Geometry: final body of the model. Coordinates: model frame, mm. Face numbers are marked on the shaded views. Give positions to 0.01 mm unless a question says otherwise; leave off trailing zeros. Write each loop counter-clockwise with the first axis right and the second up, starting at its lowest first coordinate (ties: lowest second). Pieces come first, ordered by that corner, then holes. Notation, with made-up numbers: (83, -13.5) -> (139, -13.5) arc R6 cw to (139, -3.5) -> close; hole circle Ø1 at (-7, 27.25). An arc over 180 degrees is marked (long way). Answer as a JSON object with one key per item and string values. Group by question number.
(1) Draft query along Y for the marked faces 1, 2, 3 and 4. Return one class per face: +Y half, -Y half, draft (parallel to the pull), parting line (faces both ways), or undercut.
(2) Section query C-C on y = 34.5. Output: boundary loops of the cut face in (x, z).
(3) Section query A-A on z = 131. Output: boundary loops of the cut face in (x, y), plus the area to 3 significant figures.
(4) Material intervals for probe 1 along X at (y, z) = (-4, 86.5); probe 2 along Y at (x, z) = (-101, 51); probe 3 along X at (y, z) = (22.5, 96.5), sorted ascending.
(5) Contact query for flat-ended pins moving along their axis: pin 1 Ø6 at (x, z) = (-61.93, 86.5) entering from +Y; pin 2 Ø8 at (y, z) = (8.5, 108) entering from +X; pin 3 Ø4 at (y, z) = (40.5, 87) entering from +X. Output: stop coordinate, or through.
(6) Section query B-B on x = -75. Output: boundary loops of the cut face in (y, z), plus the area to 3 significant figures.
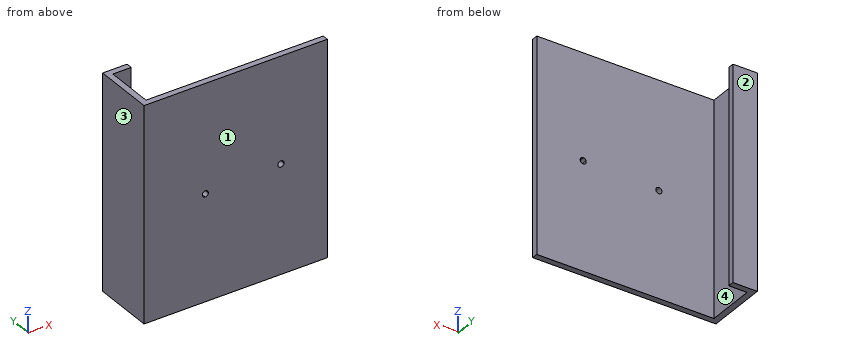
from build123d import *

# Parameters (mm, degrees)
F1_DEPTH = 175
F3_DEPTH = 25
F4_DEPTH = 25


with BuildPart() as f1:
    # F0 (on Top) → F1 (new body)
    with BuildSketch(Plane.XY):
        Polygon((-112.044677, 17.414129), (-112.044677, -7.585871), (37.955323, -7.585871), (37.955323, -2.585871), (-107.044677, -2.585871), (-107.044677, 17.414129), align=None)
        Polygon((-112.044677, 42.414129), (-112.044677, 17.414129), (-107.044677, 17.414129), (-107.044677, 37.414129), (-92.044677, 37.414129), (-92.044677, 42.414129), align=None)
    extrude(amount=F1_DEPTH)

    # F2 (on face) → F3 (cut)
    with BuildSketch(Plane.XZ.offset(7.585871)):
        with BuildLine():
            ThreePointArc((-2.327439, 89.412704), (-0.464437, 86.043519), (2.5, 88.5))
            Line((2.5, 88.5), (0, 88.5))
            Line((0, 88.5), (0, 89.526452))
            Line((0, 89.526452), (-2.327439, 89.412704))
        make_face()
    extrude(amount=-F3_DEPTH, mode=Mode.SUBTRACT)

    # F2 (on face) → F4 (cut)
    with BuildSketch(Plane.XZ.offset(7.585871)):
        with BuildLine():
            Line((0, 88.5), (2.5, 88.5))
            ThreePointArc((2.5, 88.5), (2.430881, 89.083794), (2.227347, 89.635308))
            Line((2.227347, 89.635308), (0, 89.526452))
            Line((0, 89.526452), (0, 88.5))
        make_face()
        with BuildLine():
            ThreePointArc((-59.425465, 86.5), (-59.42621, 86.561036), (-59.428445, 86.622036))
            Line((-59.428445, 86.622036), (-61.925465, 86.5))
            Line((-61.925465, 86.5), (-61.925465, 84))
            ThreePointArc((-61.925465, 84), (-60.157698, 84.732233), (-59.425465, 86.5))
        make_face()
        with BuildLine():
            Line((-61.925465, 86.5), (-59.428445, 86.622036))
            ThreePointArc((-59.428445, 86.622036), (-63.735864, 88.224081), (-61.925465, 84))
            Line((-61.925465, 84), (-61.925465, 86.5))
        make_face()
        with BuildLine():
            ThreePointArc((-2.327439, 89.412704), (-0.464437, 86.043519), (2.5, 88.5))
            Line((2.5, 88.5), (0, 88.5))
            Line((0, 88.5), (0, 89.526452))
            Line((0, 89.526452), (-2.327439, 89.412704))
        make_face()
        with BuildLine():
            Line((0, 89.526452), (2.227347, 89.635308))
            ThreePointArc((2.227347, 89.635308), (1.306088, 90.631698), (0, 91))
            Line((0, 91), (0, 89.526452))
        make_face()
        with BuildLine():
            ThreePointArc((0, 91), (-1.408588, 90.565401), (-2.327439, 89.412704))
            Line((-2.327439, 89.412704), (0, 89.526452))
            Line((0, 89.526452), (0, 91))
        make_face()
    extrude(amount=-F4_DEPTH, mode=Mode.SUBTRACT)


solid = f1.part
Answer list:
{
 "1": {"face 1": "-Y half", "face 2": "+Y half", "face 3": "draft", "face 4": "undercut"},
 "2": {"outline": "(-112.04, 0) -> (-107.04, 0) -> (-107.04, 175) -> (-112.04, 175) -> close"},
 "3": {"outline": "(-112.04, -7.59) -> (37.96, -7.59) -> (37.96, -2.59) -> (-107.04, -2.59) -> (-107.04, 37.41) -> (-92.04, 37.41) -> (-92.04, 42.41) -> (-112.04, 42.41) -> close", "area": "1,050 mm2"},
 "4": {"probe 1": "-112.04 to -64.43, -59.43 to -1.5, 1.5 to 37.96", "probe 2": "-7.59 to -2.59, 37.41 to 42.41", "probe 3": "-112.04 to -107.04"},
 "5": {"pin 1": "y = -2.59", "pin 2": "x = -107.04", "pin 3": "x = -92.04"},
 "6": {"outline": "(-7.59, 0) -> (-2.59, 0) -> (-2.59, 175) -> (-7.59, 175) -> close", "area": "875 mm2"}
}
